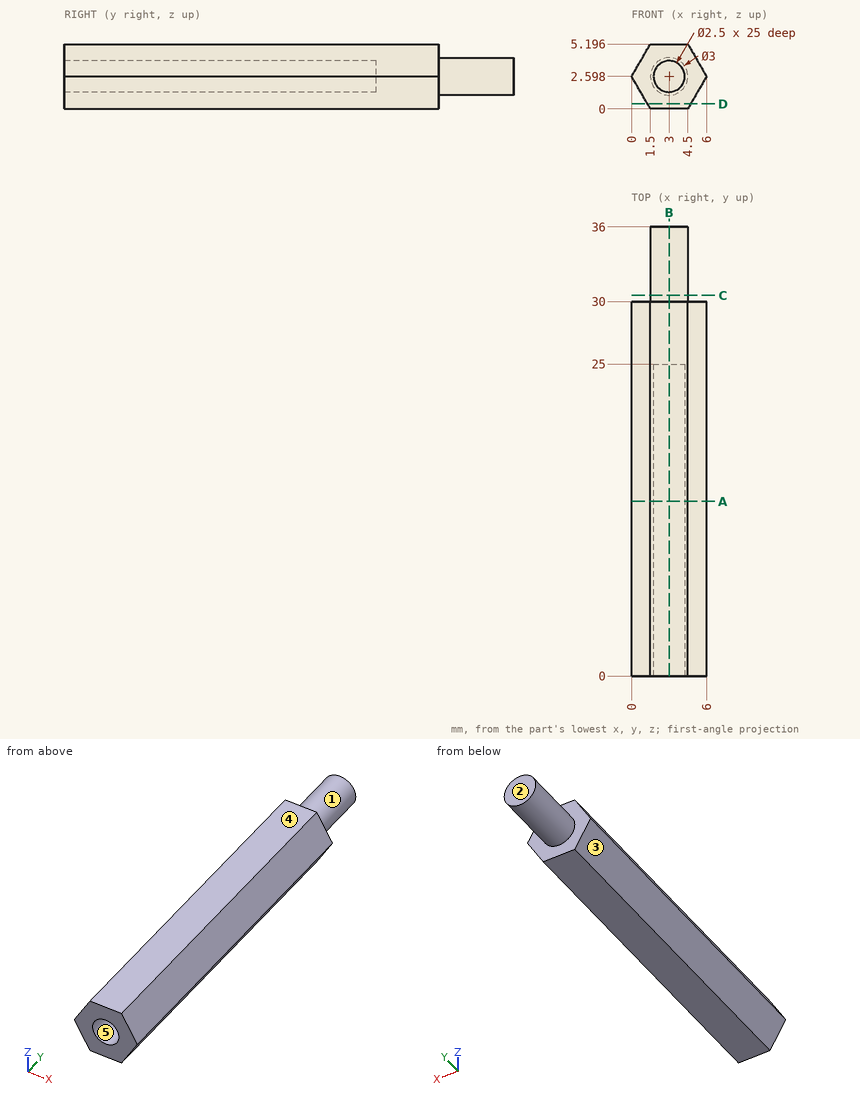
Study the drawing (mm; zero at the part's minimum x, y, z) and answer. A direction names the side the tool comes from. Coordinates: 2 decimals unless noted, no trailing zeros. Write each loop counter-clockwise with the first axis right and the second up, starting at its lowest first coordinate (ties: lowest second). Pieces come first, ordered by that corner, then holes. Notation, with made-up numbers: (50.25, 0.25) -> (94.25, 0.25) arc R25 cw to (94.25, 33.25) -> close; hole circle Ø1 at (-22, -5.75). An arc over 180 degrees is marked (long way). Write item = value, one per line.
(1) Section D-D on z = 0.4 is taken. Write down the section's boundary in (x, y), plus the area to 3 significant figures.
From the geometry:
outline = (1.27, 0) -> (4.73, 0) -> (4.73, 30) -> (1.27, 30) -> close
area = 104 mm2
(2) Section A-A on y = 14 is taken. Write down the section's boundary in (x, z).
From the geometry:
outline = (0, 2.6) -> (1.5, 0) -> (4.5, 0) -> (6, 2.6) -> (4.5, 5.2) -> (1.5, 5.2) -> close; hole circle Ø2.5 at (3, 2.6)
(3) Which of the six approach directions +Z, -Z, +X, -X, +Y, -Y give full straight-line access (tool end or side, diameter ignored) to the marked faces 1 and 2?
From the geometry:
face_1 = +Y
face_2 = +Z, -Z, +X, -X, +Y
(4) Section C-C on y = 30.5 is taken. Write down the section's boundary in (x, z), plus the area to 3 significant figures.
From the geometry:
outline = circle Ø3 at (3, 2.6)
area = 7.07 mm2
(5) For a pull along X with two mould halves and no side action, classify the marked faces 3, 4 and 5 as +X half, -X half, draft (parallel to the pull), parting line (faces both ways), or undercut.
From the geometry:
face_3 = -X half
face_4 = draft
face_5 = undercut
(6) Given pin 1 Ø1.5 at (y, z) = (30.5, 4.5) entering from -X (1 decimal); pin 2 Ø1.5 at (x, y) = (1, 32) entering from +Z, each flat-ended and moving along its own axis, determine where each tip first touches the part or whether it passes through.
From the geometry:
pin_1 = 0.8
pin_2 = 3.43
(7) Section B-B on x = 3 is taken. Write down the section's boundary in (y, z).
From the geometry:
outline = (0, 0) -> (30, 0) -> (30, 1.1) -> (36, 1.1) -> (36, 4.1) -> (30, 4.1) -> (30, 5.2) -> (0, 5.2) -> (0, 3.85) -> (25, 3.85) -> (25, 1.35) -> (0, 1.35) -> close
(8) Straight lines are drawn through the part: L1, parallel to Z at x = 3, y = 7.5; L2, parallel to Y at x = 3.15, z = 1.65; L3, parallel to Y at x = 2, z = 1.1. For each, find the intervals that lie inside material, in ascending order. Write a range as from..to.
From the geometry:
L1 = 0..1.35, 3.85..5.2
L2 = 25..36
L3 = 0..30
